from build123d import *

# Parameters (mm, degrees)
SALIENTE_EXTRUIR1_DEPTH = 13.5
CROQUIS2_R              = 2
SALIENTE_EXTRUIR2_DEPTH = 1
CROQUIS6_W              = 6
CROQUIS6_H              = 6
SALIENTE_EXTRUIR3_DEPTH = 8
CROQUIS7_W              = 6
CROQUIS7_H              = 6
SALIENTE_EXTRUIR4_DEPTH = 8
CROQUIS8_W              = 23
CROQUIS8_H              = 20
SALIENTE_EXTRUIR5_DEPTH = 16
CROQUIS9_W              = 20
CROQUIS9_H              = 17
SALIENTE_EXTRUIR6_DEPTH = 17


with BuildPart() as part:
    # Croquis1 → Saliente-Extruir1 (new body)
    with BuildSketch(Plane.XY):
        Polygon((-9.958809275, -27.124651578), (13.041190725, -27.124651578), (13.041190725, 14.875348422), (4.541190725, 14.875348422), (4.541190725, 20.875348422), (-1.458809275, 20.875348422), (-1.458809275, 14.875348422), (-9.958809275, 14.875348422), align=None)
    extrude(amount=SALIENTE_EXTRUIR1_DEPTH)

    # Croquis2 → Saliente-Extruir2 (add)
    with BuildSketch(Plane(origin=(0, 0, 0), x_dir=(-1, 0, 0), z_dir=(0, 0, -1))):
        with Locations((-1.541190725, -16.124651578)):
            Circle(CROQUIS2_R)
    extrude(amount=SALIENTE_EXTRUIR2_DEPTH)

    # Croquis6 → Saliente-Extruir3 (add)
    with BuildSketch(Plane.XY.offset(13.5)):
        with Locations((1.541190725, -8.124651578)):
            Rectangle(CROQUIS6_W, CROQUIS6_H)
    extrude(amount=SALIENTE_EXTRUIR3_DEPTH)

    # Croquis7 → Saliente-Extruir4 (add)
    with BuildSketch(Plane.XY.offset(13.5)):
        with Locations((1.541190725, 17.875348422)):
            Rectangle(CROQUIS7_W, CROQUIS7_H)
    extrude(amount=SALIENTE_EXTRUIR4_DEPTH)

    # Croquis8 → Saliente-Extruir5 (add)
    with BuildSketch(Plane.XY.offset(13.5)):
        with Locations((1.541190725, 4.875348422)):
            Rectangle(CROQUIS8_W, CROQUIS8_H)
    extrude(amount=SALIENTE_EXTRUIR5_DEPTH)

    # Croquis9 → Saliente-Extruir6 (add)
    with BuildSketch(Plane.XY.offset(29.5)):
        with Locations((1.541190725, 4.875348422)):
            Rectangle(CROQUIS9_W, CROQUIS9_H)
    extrude(amount=SALIENTE_EXTRUIR6_DEPTH)


solid = part.part
Input: part model. Units: mm. Frame: model coordinates. A direction names the side the tool comes from. Give positions to 0.01 mm unless a question says otherwise; leave off trailing zeros. Write each loop counter-clockwise with the first axis right and the second up, starting at its lowest first coordinate (ties: lowest second). Pieces come first, ordered by that corner, then holes. Notation, with made-up numbers: (88.5, 48) -> (108.5, 48) arc R17 cw to (108.5, 55) -> close; hole circle Ø3 at (79.25, 39). An arc over 180 degrees is marked (long way). Use one line per item in the form item = value. Start each with the question number.
1) Section query B-B on z = 6.5. Return the cut outline in (x, y).
2) Section query D-D on x = 1. Return the cut outline in (y, z), then the cut area to 3 significant figures.
3) Ray query, probe 1 along Z at (x, y) = (-0.5, 12); probe 2 along Y at (x, z) = (-4.5, 10.5); probe 3 along Y at (x, z) = (8.25, 19.5). Return the intervals inside material, ascending. Write a range as from..to.
4) Section query C-C on y = -9. Return the cut outline in (x, z), then the cut area to 4 significant figures.
5) Pin query (flat end, axial travel): pin 1 (6.5 mm diameter, centred on y = -9, z = 15.5, fed in from -X); pin 2 (12 mm diameter, centred on x = 3, z = 25.5, fed in from -Y); pin 3 (1 mm diameter, centred on x = 5.5, z = 18.5, fed in from -Y); pin 4 (1 mm diameter, centred on x = -7, z = 8, fed in from +Y). Return the tip coordinate at first contact, or that it passes through.
6) Set-up query: faces 1 (the flat face through (4.541, -8, 17)), 2 (the flat face through (11.541, 5, 38)), 3 (the flat face through (-1.459, -8, 17)), 4 (the flat face through (1, 18, 21.5)). Return all of +Z, -Z, +X, -X, +Y, -Y with unobstructed straight access to the full face (end or side cutting, diameter ignored); none if empty.
7) Draft query along Y for faces 5 (the flat face through (1, -11.125, 17)), 6 (the flat face through (-1.459, 18, 11)), 7 (the flat face through (1, 20.875, 11)). Return one class per face: pulls with the +Y half, pulls with the -Y half, needs draft (parallel to the pull), parting line crosses it, or undercut.
8) Section query A-A on x = 9. Return the cut outline in (y, z).
Outcome:
q1.outline = (-9.96, -27.12) -> (13.04, -27.12) -> (13.04, 14.88) -> (4.54, 14.88) -> (4.54, 20.88) -> (-1.46, 20.88) -> (-1.46, 14.88) -> (-9.96, 14.88) -> close
q2.outline = (-27.12, 0) -> (-18.05, 0) -> (-18.05, -1) -> (-14.2, -1) -> (-14.2, 0) -> (20.88, 0) -> (20.88, 21.5) -> (14.88, 21.5) -> (14.88, 29.5) -> (13.38, 29.5) -> (13.38, 46.5) -> (-3.62, 46.5) -> (-3.62, 29.5) -> (-5.12, 29.5) -> (-5.12, 21.5) -> (-11.12, 21.5) -> (-11.12, 13.5) -> (-27.12, 13.5) -> close
q2.area = 1,360 mm^2
q3.probe_1 = 0..46.5
q3.probe_2 = -27.12..14.88
q3.probe_3 = -5.12..14.88
q4.outline = (-9.96, 0) -> (13.04, 0) -> (13.04, 13.5) -> (4.54, 13.5) -> (4.54, 21.5) -> (-1.46, 21.5) -> (-1.46, 13.5) -> (-9.96, 13.5) -> close
q4.area = 358.5 mm^2
q5.pin_1 = -9.96
q5.pin_2 = -11.12
q5.pin_3 = -5.12
q5.pin_4 = 14.88
q6.face_1 = +Z, +X, -Y
q6.face_2 = +Z, +X, +Y, -Y
q6.face_3 = +Z, -X, -Y
q6.face_4 = +Z, +X, -X, +Y
q7.face_5 = pulls with the -Y half
q7.face_6 = needs draft
q7.face_7 = pulls with the +Y half
q8.outline = (-27.12, 0) -> (14.88, 0) -> (14.88, 29.5) -> (13.38, 29.5) -> (13.38, 46.5) -> (-3.62, 46.5) -> (-3.62, 29.5) -> (-5.12, 29.5) -> (-5.12, 13.5) -> (-27.12, 13.5) -> close
